Verification items for the finished model (mm, model axes). A direction names the side the tool comes from. Round coordinates to 2 decimals unless told otherwise and drop trailing zeros. Write each loop counter-clockwise with the first axis right and the second up, starting at its lowest first coordinate (ties: lowest second). Pieces come first, ordered by that corner, then holes. Notation, with made-up numbers: (6.25, 62) - (48.25, 62) arc R31 ccw to (48.25, 92) - close; hole circle Ø2 at (-27.75, -38.5). An arc over 180 degrees is marked (long way). Answer as a JSON object with one key per item and string values.
```python
from build123d import *

# Parameters (mm, degrees)
F0_W      = 88.5811836569
F0_H      = 6.35
F1_DEPTH  = 2.54
F2_START  = 67.31
F2_DEPTH  = 2.54
F3_DEPTH  = 69.85
F4_W      = 90.1380174519
F4_H      = 3.175
F5_DEPTH  = 5.08
F6_W      = 90.1380174519
F6_H      = 3.175
F7_DEPTH  = 5.08
F8_W      = 54.61
F8_H      = 3.175
F9_DEPTH  = 5.08
F10_W     = 54.61
F10_H     = 3.175
F11_DEPTH = 5.08


with BuildPart() as f1:
    # F0 (on Front) → F1 (new body)
    with BuildSketch(Plane.XZ):
        with BuildLine():
            Line((-53.1805918284, 0), (-46.8305918284, 0))
            Line((-46.8305918284, 0), (-46.8305918284, 2.54))
            Line((-46.8305918284, 2.54), (-51.160757232, 2.54))
            ThreePointArc((-51.160757232, 2.54), (-52.1861301587, 1.2822904776), (-53.1805918284, 0))
        make_face()
        with BuildLine():
            Line((46.8305918284, 2.54), (46.8305918284, 0))
            Line((46.8305918284, 0), (53.1805918284, 0))
            ThreePointArc((53.1805918284, 0), (52.1861301587, 1.2822904776), (51.160757232, 2.54))
            Line((51.160757232, 2.54), (46.8305918284, 2.54))
        make_face()
        with BuildLine():
            Line((-46.8305918284, 0), (-44.2905918284, 0))
            Line((-44.2905918284, 0), (-44.2905918284, 6.35))
            Line((-44.2905918284, 6.35), (-44.2905918284, 9.6220642611))
            ThreePointArc((-44.2905918284, 9.6220642611), (-45.5761135004, 8.4492711462), (-46.8305918284, 7.2433301096))
            Line((-46.8305918284, 7.2433301096), (-46.8305918284, 2.54))
            Line((-46.8305918284, 2.54), (-46.8305918284, 0))
        make_face()
        with BuildLine():
            Line((44.2905918284, 6.35), (44.2905918284, 0))
            Line((44.2905918284, 0), (46.8305918284, 0))
            Line((46.8305918284, 0), (46.8305918284, 2.54))
            Line((46.8305918284, 2.54), (46.8305918284, 7.2433301096))
            ThreePointArc((46.8305918284, 7.2433301096), (45.5761135004, 8.4492711462), (44.2905918284, 9.6220642611))
            Line((44.2905918284, 9.6220642611), (44.2905918284, 6.35))
        make_face()
        with Locations((0, 3.175)):
            Rectangle(F0_W, F0_H)
        with BuildLine():
            Line((-51.160757232, 2.54), (-46.8305918284, 2.54))
            Line((-46.8305918284, 2.54), (-46.8305918284, 7.2433301096))
            ThreePointArc((-46.8305918284, 7.2433301096), (-49.0520789692, 4.9435943357), (-51.160757232, 2.54))
        make_face()
        with BuildLine():
            Line((46.8305918284, 7.2433301096), (46.8305918284, 2.54))
            Line((46.8305918284, 2.54), (51.160757232, 2.54))
            ThreePointArc((51.160757232, 2.54), (49.0520789692, 4.9435943357), (46.8305918284, 7.2433301096))
        make_face()
        with BuildLine():
            Line((-44.2905918284, 6.35), (44.2905918284, 6.35))
            Line((44.2905918284, 6.35), (44.2905918284, 9.6220642611))
            ThreePointArc((44.2905918284, 9.6220642611), (23.6913300639, 22.1072974627), (0, 26.4583333333))
            ThreePointArc((0, 26.4583333333), (-23.6913300639, 22.1072974627), (-44.2905918284, 9.6220642611))
            Line((-44.2905918284, 9.6220642611), (-44.2905918284, 6.35))
        make_face()
    extrude(amount=F1_DEPTH)



with BuildPart() as f2:
    # F0 (on Front) → F2 (new body)
    with BuildSketch(Plane.XZ.offset(F2_START)):
        with BuildLine():
            Line((-53.1805918284, 0), (-46.8305918284, 0))
            Line((-46.8305918284, 0), (-46.8305918284, 2.54))
            Line((-46.8305918284, 2.54), (-51.160757232, 2.54))
            ThreePointArc((-51.160757232, 2.54), (-52.1861301587, 1.2822904776), (-53.1805918284, 0))
        make_face()
        with BuildLine():
            Line((-51.160757232, 2.54), (-46.8305918284, 2.54))
            Line((-46.8305918284, 2.54), (-46.8305918284, 7.2433301096))
            ThreePointArc((-46.8305918284, 7.2433301096), (-49.0520789692, 4.9435943357), (-51.160757232, 2.54))
        make_face()
        with BuildLine():
            Line((-46.8305918284, 0), (-44.2905918284, 0))
            Line((-44.2905918284, 0), (-44.2905918284, 6.35))
            Line((-44.2905918284, 6.35), (-44.2905918284, 9.6220642611))
            ThreePointArc((-44.2905918284, 9.6220642611), (-45.5761135004, 8.4492711462), (-46.8305918284, 7.2433301096))
            Line((-46.8305918284, 7.2433301096), (-46.8305918284, 2.54))
            Line((-46.8305918284, 2.54), (-46.8305918284, 0))
        make_face()
        with Locations((0, 3.175)):
            Rectangle(F0_W, F0_H)
        with BuildLine():
            Line((44.2905918284, 6.35), (44.2905918284, 0))
            Line((44.2905918284, 0), (46.8305918284, 0))
            Line((46.8305918284, 0), (46.8305918284, 2.54))
            Line((46.8305918284, 2.54), (46.8305918284, 7.2433301096))
            ThreePointArc((46.8305918284, 7.2433301096), (45.5761135004, 8.4492711462), (44.2905918284, 9.6220642611))
            Line((44.2905918284, 9.6220642611), (44.2905918284, 6.35))
        make_face()
        with BuildLine():
            Line((46.8305918284, 7.2433301096), (46.8305918284, 2.54))
            Line((46.8305918284, 2.54), (51.160757232, 2.54))
            ThreePointArc((51.160757232, 2.54), (49.0520789692, 4.9435943357), (46.8305918284, 7.2433301096))
        make_face()
        with BuildLine():
            Line((46.8305918284, 2.54), (46.8305918284, 0))
            Line((46.8305918284, 0), (53.1805918284, 0))
            ThreePointArc((53.1805918284, 0), (52.1861301587, 1.2822904776), (51.160757232, 2.54))
            Line((51.160757232, 2.54), (46.8305918284, 2.54))
        make_face()
        with BuildLine():
            Line((-44.2905918284, 6.35), (44.2905918284, 6.35))
            Line((44.2905918284, 6.35), (44.2905918284, 9.6220642611))
            ThreePointArc((44.2905918284, 9.6220642611), (23.6913300639, 22.1072974627), (0, 26.4583333333))
            ThreePointArc((0, 26.4583333333), (-23.6913300639, 22.1072974627), (-44.2905918284, 9.6220642611))
            Line((-44.2905918284, 9.6220642611), (-44.2905918284, 6.35))
        make_face()
    extrude(amount=F2_DEPTH)


with BuildPart() as f1_1:
    add(f1.part)

    add(f2.part)  # F3 merges F2
    # F0 (on Front) → F3 (join)
    with BuildSketch(Plane.XZ):
        with BuildLine():
            Line((-46.8305918284, 0), (-44.2905918284, 0))
            Line((-44.2905918284, 0), (-44.2905918284, 6.35))
            Line((-44.2905918284, 6.35), (-44.2905918284, 9.6220642611))
            ThreePointArc((-44.2905918284, 9.6220642611), (-45.5761135004, 8.4492711462), (-46.8305918284, 7.2433301096))
            Line((-46.8305918284, 7.2433301096), (-46.8305918284, 2.54))
            Line((-46.8305918284, 2.54), (-46.8305918284, 0))
        make_face()
        with BuildLine():
            Line((44.2905918284, 6.35), (44.2905918284, 0))
            Line((44.2905918284, 0), (46.8305918284, 0))
            Line((46.8305918284, 0), (46.8305918284, 2.54))
            Line((46.8305918284, 2.54), (46.8305918284, 7.2433301096))
            ThreePointArc((46.8305918284, 7.2433301096), (45.5761135004, 8.4492711462), (44.2905918284, 9.6220642611))
            Line((44.2905918284, 9.6220642611), (44.2905918284, 6.35))
        make_face()
    extrude(amount=F3_DEPTH)

    # F4 (on face) → F5 (join)
    with BuildSketch(Plane.XZ.offset(2.54)):
        with Locations((0.7784168975, 1.5875)):
            Rectangle(F4_W, F4_H)
    extrude(amount=F5_DEPTH)

    # F6 (on face) → F7 (join)
    with BuildSketch(Plane(origin=(0, -67.31, 0), x_dir=(-1, 0, 0), z_dir=(0, 1, 0))):
        with Locations((0.7784168975, 1.5875)):
            Rectangle(F6_W, F6_H)
    extrude(amount=F7_DEPTH)

    # F8 (on face) → F9 (join)
    with BuildSketch(Plane.YZ.offset(-44.2905918284)):
        with Locations((-34.925, 1.5875)):
            Rectangle(F8_W, F8_H)
    extrude(amount=F9_DEPTH)

    # F10 (on face) → F11 (join)
    with BuildSketch(Plane(origin=(44.2905918284, 0, 0), x_dir=(0, -1, 0), z_dir=(-1, 0, 0))):
        with Locations((34.925, 1.5875)):
            Rectangle(F10_W, F10_H)
    extrude(amount=F11_DEPTH)


solid = f1_1.part
```
1. Access from +Z, -Z, +X, -X, +Y, -Y to the whole of each face (thin tool, end or side, straight path). Record for faces 1 (the face through (-49, -67.31, 3)), 2 (the face through (49, -2.54, 3)), 3 (the face through (8, -6, 0)), 4 (the face through (39.211, -35, 2)), 5 (the face through (-1, -67.31, 12)).
Completed:
{"face 1": "+Z, -Z, -X", "face 2": "+Z, -Z, +X", "face 3": "-Z, +X, -X, +Y, -Y", "face 4": "+Z, -Z", "face 5": "+Z"}
2. Go/stop test with flat-tipped pins: pin 1 (3.5 mm diameter, centred on y = -38.5, z = 2.5, fed in from +X); pin 2 (8 mm diameter, centred on y = -37, z = 3, fed in from -X); pin 3 (2 mm diameter, centred on y = -45.5, z = 10.5, fed in from -X); pin 4 (4 mm diameter, centred on x = 27.5, y = -10, fed in from +Z). Record where each tip stops, or that it passes through.
Completed:
{"pin 1": "stops at x = 46.83", "pin 2": "stops at x = -46.83", "pin 3": "stops at x = -44.43", "pin 4": "passes through"}
3. Material ranges on probe 1 along Y at (x, z) = (-11, 1); probe 2 along Y at (x, z) = (15, 22); probe 3 along X at (y, z) = (-12.5, 3), recorded low to high. Write a range as from..to.
Completed:
{"probe 1": "y = -69.85..-62.23, -7.62..0", "probe 2": "y = -69.85..-67.31, -2.54..0", "probe 3": "x = -46.83..-39.21, 39.21..46.83"}
4. Cross-section at B-B (z = 16.5). Record the boundary of the cut face in (x, y), plus the area to 3 significant figures.
Completed:
{"outline": "(-35.05, -69.85) - (35.05, -69.85) - (35.05, -67.31) - (-35.05, -67.31) - close; (-35.05, -2.54) - (35.05, -2.54) - (35.05, 0) - (-35.05, 0) - close", "area": "356 mm^2"}
5. Cross-section at D-D (z = 5.75). Record the boundary of the cut face in (x, y), plus the area to 3 significant figures.
Completed:
{"outline": "(-48.3, -69.85) - (48.3, -69.85) - (48.3, -67.31) - (46.83, -67.31) - (46.83, -2.54) - (48.3, -2.54) - (48.3, 0) - (-48.3, 0) - (-48.3, -2.54) - (-46.83, -2.54) - (-46.83, -67.31) - (-48.3, -67.31) - close; hole (-44.29, -67.31) - (44.29, -67.31) - (44.29, -2.54) - (-44.29, -2.54) - close", "area": "820 mm^2"}
6. Cross-section at A-A (y = -13.5). Record the boundary of the cut face in (x, z) (3 decimals), plus the area to 3 significant figures.
Completed:
{"outline": "(-46.831, 0) - (-39.211, 0) - (-39.211, 3.175) - (-44.291, 3.175) - (-44.291, 9.622) arc R66.675 ccw to (-46.831, 7.243) - close; (39.211, 0) - (46.831, 0) - (46.831, 7.243) arc R66.675 ccw to (44.291, 9.622) - (44.291, 3.175) - (39.211, 3.175) - close", "area": "75.2 mm^2"}
7. Mould release check, pull along Y, two halves, no side actions. Record for faces 6 (the face through (-1, -69.85, 10)), 7 (the face through (-1, 0, 10)), 8 (the face through (44.291, -34, 6)), 9 (the face through (-44.291, -34, 6)): released by +Y, released by -Y, zero draft, split by the parting line, or undercut.
Completed:
{"face 6": "released by -Y", "face 7": "released by +Y", "face 8": "undercut", "face 9": "undercut"}
8. Cross-section at C-C (x = -7.5). Record the boundary of the cut face in (y, z) (3 decimals), plus the area to 3 significant figures.
Completed:
{"outline": "(-69.85, 0) - (-62.23, 0) - (-62.23, 3.175) - (-67.31, 3.175) - (-67.31, 26.035) - (-69.85, 26.035) - close; (-7.62, 0) - (0, 0) - (0, 26.035) - (-2.54, 26.035) - (-2.54, 3.175) - (-7.62, 3.175) - close", "area": "165 mm^2"}
